The listing builds one solid part. Answer for the finished solid, in the listing's coordinates (mm). A direction names the side the tool comes from. Round coordinates to 2 decimals unless told otherwise and drop trailing zeros. Write each loop counter-clockwise with the first axis right and the second up, starting at its lowest first coordinate (ties: lowest second). Pieces come first, ordered by that corner, then holes. Notation, with made-up numbers: M 4,74.5 L 42,74.5 A14 cw 42,87.5 Z; hole C 86,65 d8. An arc over 180 degrees is marked long. One line per item, written item: value. Start each with the question number.
(1) For a pull along Z with two mould halves and no side action, classify faces 6 (the flat face through (-28, 7.525, -53)), 7 (the flat face through (-28, -1, -57.35)), 8 (the flat face through (-53, 7.525, -28)) as released by +Z, released by -Z, zero draft, split by the parting line, or undercut.
(2) Section C-C (z = -27) is taken. Determine the outline of the cut face in (x, y) (3 decimals).
(3) Consider probe 1 along Z at (x, y) = (4.5, -7.5); probe 2 along X at (y, z) = (10.25, 52.5); probe 3 along X at (y, z) = (-8.75, -58). Determine where each line is inside the solid, lowest interval first.
(4) Section D-D (x = -53.5) is taken. Determine the outline of the cut face in (y, z) (3 decimals), plus the area to 3 significant figures.
(5) Given P1, Ø1.5, axis at x = 14, z = 8.5, coming from the +Y side; P2, Ø1, axis at x = 35, y = -6.5, coming from the +Z side; P3, Ø10.5, axis at x = -28, z = -53.5, coming from the +Y side; P4, Ø1.5, axis at y = 3.5, z = 29.5, coming from the +X side, each flat-ended and moving along its own axis, determine where each tip first touches the part or whether it passes through.
(6) Section A-A (x = 29.5) is taken. Determine the outline of the cut face in (y, z) (3 decimals).
(7) For faces 1 (the flat face through (0, 12.4, 58)), 2 (the flat face through (-43, -11, -38)), 3 (the flat face through (-54, 10, 33.363)), 4 (the flat face through (23.203, 10, -54)), 5 (the flat face through (64, -9.7, 28)), determine the directions among +Z, -Z, +X, -X, +Y, -Y from which every point of the face is accessible in a straight line to the end or side of a thin tool.
(8) Section B-B (z = 38) is taken. Determine the outline of the cut face in (x, y), plus the area to 3 significant figures.
```python
from build123d import *

# Parameters (mm, degrees)
SKETCH1_W           = 139.7
SKETCH1_H           = 139.7
BOSS_EXTRUDE1_DEPTH = 12.7
SKETCH2_W           = 139.7
SKETCH2_H           = 139.7
CUT_EXTRUDE1_DEPTH  = 0.3
CUT_EXTRUDE2_START  = -22.1
CUT_EXTRUDE2_DEPTH  = 125.021808265
SKETCH18_W          = 10.16
SKETCH18_H          = 4.875
CUT_EXTRUDE6_DEPTH  = 20
CIRPATTERN1_COUNT   = 4
SKETCH19_W          = 100
SKETCH19_H          = 100
CUT_EXTRUDE8_DEPTH  = 3.5
SKETCH20_W          = 96
SKETCH20_H          = 96
CUT_EXTRUDE9_DEPTH  = 18.6
SKETCH21_W          = 30
SKETCH21_H          = 10
CUT_EXTRUDE10_DEPTH = 102.224774635
FILLET2_R           = 1.5
CIRPATTERN2_COUNT   = 2


with BuildPart() as part:
    # Sketch1 → Boss-Extrude1 (new, symmetric)
    with BuildSketch(Plane(origin=(0, 0, 0), x_dir=(1, 0, 0), z_dir=(0, 1, 0))):
        Rectangle(SKETCH1_W, SKETCH1_H)
    extrude(amount=BOSS_EXTRUDE1_DEPTH, both=True)

    # Sketch2 → Cut-Extrude1 (cut)
    with BuildSketch(Plane(origin=(0, 12.7, 0), x_dir=(1, 0, 0), z_dir=(0, 1, 0))):
        Rectangle(SKETCH2_W, SKETCH2_H)
    extrude(amount=-CUT_EXTRUDE1_DEPTH, mode=Mode.SUBTRACT)

    # Sketch4 → Cut-Extrude2 (cut)
    with BuildSketch(Plane(origin=(0, 12.4, 0), x_dir=(1, 0, 0), z_dir=(0, 1, 0)).offset(CUT_EXTRUDE2_START)):
        Polygon((-43.283333333, -69.85), (-50.500211698, -57.35), (-6.066454968, -57.35), (-13.283333333, -69.85), align=None)
        Polygon((43.283333333, -69.85), (36.066454968, -57.35), (20.500211698, -57.35), (13.283333333, -69.85), align=None)
    cut_extrude2 = extrude(amount=CUT_EXTRUDE2_DEPTH, mode=Mode.SUBTRACT)

    # Sketch18 → Cut-Extrude6 (cut)
    with BuildSketch(Plane.XY.offset(57.35)):
        with Locations((28.283333333, 9.9625)):
            Rectangle(SKETCH18_W, SKETCH18_H)
        with Locations((-28.283333333, 9.9625)):
            Rectangle(SKETCH18_W, SKETCH18_H)
    cut_extrude6 = extrude(amount=-CUT_EXTRUDE6_DEPTH, mode=Mode.SUBTRACT)

    # CirPattern1: Cut-Extrude2, Cut-Extrude6 ×4 about axis
    cirpattern1_axis = Axis((0, 0, 0), (0, 1, 0))
    add([cut_extrude2.rotate(cirpattern1_axis, i * 360 / CIRPATTERN1_COUNT) for i in range(1, CIRPATTERN1_COUNT)], mode=Mode.SUBTRACT)
    add([cut_extrude6.rotate(cirpattern1_axis, i * 360 / CIRPATTERN1_COUNT) for i in range(1, CIRPATTERN1_COUNT)], mode=Mode.SUBTRACT)

    # Sketch19 → Cut-Extrude8 (cut)
    with BuildSketch(Plane(origin=(0, 12.4, 0), x_dir=(1, 0, 0), z_dir=(0, 1, 0))):
        Rectangle(SKETCH19_W, SKETCH19_H)
    extrude(amount=-CUT_EXTRUDE8_DEPTH, mode=Mode.SUBTRACT)

    # Sketch20 → Cut-Extrude9 (cut)
    with BuildSketch(Plane(origin=(0, 8.9, 0), x_dir=(1, 0, 0), z_dir=(0, 1, 0))):
        Rectangle(SKETCH20_W, SKETCH20_H)
    extrude(amount=-CUT_EXTRUDE9_DEPTH, mode=Mode.SUBTRACT)

    # Sketch21 → Cut-Extrude10 (cut, through all)
    with BuildSketch(Plane(origin=(0, -9.7, 0), x_dir=(1, 0, 0), z_dir=(0, 1, 0))):
        with Locations((-28, 38)):
            Rectangle(SKETCH21_W, SKETCH21_H)
    cut_extrude10 = extrude(amount=-CUT_EXTRUDE10_DEPTH, mode=Mode.SUBTRACT)

    # Fillet2
    fillet2_edges = [part.edges().sort_by_distance(p)[0] for p in [
        (50, 10.65, 50),
        (-50, 10.65, -50),
        (50, 10.65, -50),
        (-50, 10.65, 50),
        (48, -0.4, -48),
        (48, -0.4, 48),
        (-48, -0.4, 48),
        (-48, -0.4, -48),
    ]]
    fillet(fillet2_edges, radius=FILLET2_R)

    # CirPattern2: Cut-Extrude10 ×2 about axis
    cirpattern2_axis = Axis((0, 0, 0), (0, 1, 0))
    for i in range(1, CIRPATTERN2_COUNT):
        add(cut_extrude10.rotate(cirpattern2_axis, i * 360 / CIRPATTERN2_COUNT), mode=Mode.SUBTRACT)


solid = part.part
```
Recorded:
1. face 6: zero draft
1. face 7: released by -Z
1. face 8: undercut
2. outline: M -69.85,-12.7 L 69.85,-12.7 L 69.85,-9.7 L 57.35,-9.7 L 57.35,7.525 L 48,7.525 L 48,-9.7 L -48,-9.7 L -48,7.525 L -57.35,7.525 L -57.35,-9.7 L -69.85,-9.7 Z
3. probe 1: z = -69.85 to -48, 48 to 69.85
3. probe 2: x = -69.85 to -33.36, -23.2 to 23.2, 33.36 to 69.85
3. probe 3: x = -69.85 to -36.44, -20.12 to 6.44, 50.12 to 69.85
4. outline: M -12.7,-69.85 L 12.4,-69.85 L 12.4,-33.363 L 7.525,-33.363 L 7.525,-23.203 L 12.4,-23.203 L 12.4,23.203 L 7.525,23.203 L 7.525,33.363 L 12.4,33.363 L 12.4,69.85 L -12.7,69.85 Z
4. area: 3,410 mm2
5. P1: stops at y = -9.7
5. P2: stops at z = 57.35
5. P3: stops at y = 12.4
5. P4: stops at x = 57.35
6. outline: M -12.7,-69.85 L -9.7,-69.85 L -9.7,-57.35 L 7.525,-57.35 L 7.525,-48 L -9.7,-48 L -9.7,33 L -12.7,33 Z; M -12.7,43 L -9.7,43 L -9.7,48 L 7.525,48 L 7.525,57.35 L -9.7,57.35 L -9.7,69.85 L -12.7,69.85 Z
7. face 1: +Z, -Z, +X, -X, +Y
7. face 2: +Y, -Y
7. face 3: +X, -X, +Y
7. face 4: +Z, -Z, +Y
7. face 5: +Y
8. outline: M -69.85,-12.7 L 13,-12.7 L 13,-9.7 L -48,-9.7 L -48,8.9 L -50,8.9 L -50,12.4 L -60.7,12.4 L -60.7,-9.7 L -69.85,-9.7 Z; M 43,-12.7 L 69.85,-12.7 L 69.85,-9.7 L 57.35,-9.7 L 57.35,12.4 L 50,12.4 L 50,8.9 L 48,8.9 L 48,-9.7 L 43,-9.7 Z
8. area: 802 mm2
